from build123d import *

# Parameters (mm, degrees)
BOSS_EXTRUDE1_DEPTH     = 9.525
SKETCH12_R              = 2.75
CUT_EXTRUDE2_DEPTH      = 236.564695201
CUT_EXTRUDE3_DEPTH      = 289.081109455
CUT_EXTRUDE3_DEPTH_BACK = 289.081109455
SKETCH13_R              = 2.75
CUT_EXTRUDE6_REACH      = 237.565
SKETCH16_R              = 2.75
CUT_EXTRUDE7_DEPTH      = 289.081109455
CUT_EXTRUDE7_DEPTH_BACK = 289.081109455
SKETCH17_R              = 3


with BuildPart() as part:
    # Sketch1 → Boss-Extrude1 (new, symmetric)
    with BuildSketch(Plane.XY):
        with BuildLine():
            Line((50, 45), (50, 240))
            ThreePointArc((50, 240), (41.213203436, 261.213203436), (20, 270))
            Line((20, 270), (-20, 270))
            ThreePointArc((-20, 270), (-41.213203436, 261.213203436), (-50, 240))
            Line((-50, 240), (-50, 45))
            ThreePointArc((-50, 45), (-48.535533906, 41.464466094), (-45, 40))
            Line((-45, 40), (-31.825, 40))
            Line((-31.825, 40), (-31.825, 43.175))
            Line((-31.825, 43.175), (-45, 43.175))
            ThreePointArc((-45, 43.175), (-46.290469876, 43.709530124), (-46.825, 45))
            Line((-46.825, 45), (-46.825, 240))
            ThreePointArc((-46.825, 240), (-38.968139405, 258.968139405), (-20, 266.825))
            Line((-20, 266.825), (20, 266.825))
            ThreePointArc((20, 266.825), (38.968139405, 258.968139405), (46.825, 240))
            Line((46.825, 240), (46.825, 45))
            ThreePointArc((46.825, 45), (46.290469876, 43.709530124), (45, 43.175))
            Line((45, 43.175), (31.825, 43.175))
            Line((31.825, 43.175), (31.825, 40))
            Line((31.825, 40), (45, 40))
            ThreePointArc((45, 40), (48.535533906, 41.464466094), (50, 45))
        make_face()
    extrude(amount=BOSS_EXTRUDE1_DEPTH, both=True)

    # Sketch12 → Cut-Extrude2 (cut, through all)
    with BuildSketch(Plane(origin=(0, 270, 0), x_dir=(1, 0, 0), z_dir=(0, 1, 0))):
        with Locations(Location((0, 0, 0), (0, 0, 270))):
            Circle(SKETCH12_R)
        with Locations(Location((-15, 0, 0), (0, 0, 270))):
            Circle(SKETCH12_R)
        with Locations(Location((15, 0, 0), (0, 0, 270))):
            Circle(SKETCH12_R)
    extrude(amount=-CUT_EXTRUDE2_DEPTH, mode=Mode.SUBTRACT)

    # Sketch13 → Cut-Extrude3 (cut, two sides: drawn at the far end of the back side and taken through both)
    with BuildSketch(Plane(origin=(50, 0, 0), x_dir=(0, 0, -1), z_dir=(1, 0, 0)).offset(-CUT_EXTRUDE3_DEPTH_BACK)):
        with Locations(Location((0, 205, 0), (0, 0, 90))):
            Circle(SKETCH13_R)
        with Locations(Location((0, 140, 0), (0, 0, 90))):
            Circle(SKETCH13_R)
        with Locations(Location((0, 75, 0), (0, 0, 90))):
            Circle(SKETCH13_R)
    extrude(amount=CUT_EXTRUDE3_DEPTH + CUT_EXTRUDE3_DEPTH_BACK, mode=Mode.SUBTRACT)

    # Sketch16 → Cut-Extrude6 (cut, up to next)
    with BuildSketch(Plane(origin=(0, 40, 0), x_dir=(-1, 0, 0), z_dir=(0, -1, 0)), mode=Mode.PRIVATE) as cut_extrude6_sk1:
        with Locations(Location((38.4125, 0, 0), (0, 0, 180))):
            Circle(SKETCH16_R)
    cut_extrude6_tool1 = extrude(cut_extrude6_sk1.sketch, amount=-CUT_EXTRUDE6_REACH, mode=Mode.PRIVATE) & part.part
    # Sketch16 → Cut-Extrude6 (cut, up to next)
    with BuildSketch(Plane(origin=(0, 40, 0), x_dir=(-1, 0, 0), z_dir=(0, -1, 0)), mode=Mode.PRIVATE) as cut_extrude6_sk2:
        with Locations(Location((-38.4125, 0, 0), (0, 0, 180))):
            Circle(SKETCH16_R)
    cut_extrude6_tool2 = extrude(cut_extrude6_sk2.sketch, amount=-CUT_EXTRUDE6_REACH, mode=Mode.PRIVATE) & part.part
    add(cut_extrude6_tool1.solids().sort_by_distance((-38.4125, 40, 0))[0], mode=Mode.SUBTRACT)
    add(cut_extrude6_tool2.solids().sort_by_distance((38.4125, 40, 0))[0], mode=Mode.SUBTRACT)

    # Sketch17 → Cut-Extrude7 (cut, two sides: drawn at the far end of the back side and taken through both)
    with BuildSketch(Plane(origin=(50, 0, 0), x_dir=(0, 0, -1), z_dir=(1, 0, 0)).offset(-CUT_EXTRUDE7_DEPTH_BACK)):
        with Locations(Location((0, 220, 0), (0, 0, 90))):
            Circle(SKETCH17_R)
    extrude(amount=CUT_EXTRUDE7_DEPTH + CUT_EXTRUDE7_DEPTH_BACK, mode=Mode.SUBTRACT)


solid = part.part
Input: part model. Units: mm. Frame: model coordinates. A direction names the side the tool comes from. Coordinates: 2 decimals unless noted, no trailing zeros. Write each loop counter-clockwise with the first axis right and the second up, starting at its lowest first coordinate (ties: lowest second). Pieces come first, ordered by that corner, then holes. Notation, with made-up numbers: M 68.5,1 L 88.5,1 A30 ccw 88.5,36 Z; hole C 70.5,81.25 d2. An arc over 180 degrees is marked long. Answer as a JSON object with one key per item and string values. Group by question number.
(1) Section D-D on z = 0. Give the number of separate pieces and of enclosed holes in the cut face, plus the area to 3 significant figures.
(2) Ray query, line 1 along X through (y, z) = (207, 3.5) (3 decimals); line 2 along Y through (x, z) = (-19, 3.25) (3 decimals); line 3 along Y through (x, z) = (33.5, -5.5) (3 decimals). Return the intervals inside material, ascending. Write a range as [from, to].
(3) Set-up query: faces 1 (the face through (41.445, 260.979, 0.133)), 2 (the face through (46.825, 144, 0)). Return all of +Z, -Z, +X, -X, +Y, -Y with unobstructed straight access to the full face (end or side cutting, diameter ignored); none if empty.
(4) Mould query, pull axis Y, two halves, no side actions, for faces 3 (the face through (-12.273, 268.435, -0.358)), 4 (the face through (0, 270, 4)), 5 (the face through (48.39, 207.62, 0.83)), 6 (the face through (48, 217, 0)). Classes: pulls with the +Y half, pulls with the -Y half, needs draft (parallel to the pull), parting line crosses it, or undercut.
(5) Section C-C on y = 114. Output: boundary loops of the cut face in (x, z) (3 decimals), plus the area to 3 significant figures.
(6) Section A-A on x = 15. Output: boundary loops of the cut face in (y, z) (3 decimals), plus the area to 3 significant figures.
(7) Section B-B on y = 75. Output: boundary loops of the cut face in (x, z) (3 decimals).
(8) Contact query for flat-ended pins moving along their axis: P1, Ø4.5, axis at x = 15, z = 0, coming from the -Y side; P2, Ø5, axis at x = 38.41, z = 0, coming from the +Y side; P3, Ø5.5, axis at x = -8.5, z = 4, coming from the -Y side (3 decimals); P4, Ø10.5, axis at x = 38.5, z = -3, coming from the +Y side. Output: stop coordinate, or through.
Result set:
{
 "1": {"separate pieces": "14", "enclosed holes": "0", "area": "1,540 mm2"},
 "2": {"line 1": "x = [-50, -46.825], [46.825, 50]", "line 2": "y = [266.825, 270]", "line 3": "y = [40, 43.175], [263.18, 266.791]"},
 "3": {"face 1": "+Z, -Z, +X, +Y", "face 2": "+Z, -Z"},
 "4": {"face 3": "needs draft", "face 4": "pulls with the +Y half", "face 5": "undercut", "face 6": "undercut"},
 "5": {"outline": "M -50,-9.525 L -46.825,-9.525 L -46.825,9.525 L -50,9.525 Z; M 46.825,-9.525 L 50,-9.525 L 50,9.525 L 46.825,9.525 Z", "area": "121 mm2"},
 "6": {"outline": "M 266.825,-9.525 L 270,-9.525 L 270,-2.75 L 266.825,-2.75 Z; M 266.825,2.75 L 270,2.75 L 270,9.525 L 266.825,9.525 Z", "area": "43.0 mm2"},
 "7": {"outline": "M -50,-9.525 L -46.825,-9.525 L -46.825,-2.75 L -50,-2.75 Z; M -50,2.75 L -46.825,2.75 L -46.825,9.525 L -50,9.525 Z; M 46.825,-9.525 L 50,-9.525 L 50,-2.75 L 46.825,-2.75 Z; M 46.825,2.75 L 50,2.75 L 50,9.525 L 46.825,9.525 Z"},
 "8": {"P1": "passes through", "P2": "stops at y = 265.43", "P3": "stops at y = 266.825", "P4": "stops at y = 266.92"}
}
